Check sheet for the modelled part. Datum: model origin and axes. Units: mm. A direction names the side the tool comes from. Give positions to 0.01 mm unless a question says otherwise; leave off trailing zeros. Order: outer loops, then holes, each group sorted by start corner. A loop starts at its lowest first (then second) coordinate and runs counter-clockwise, first axis right, second up. Notation, with made-up numbers: (87.25, -13.5) -> (118.25, -13.5) arc R27 cw to (118.25, 4.5) -> close; hole circle Ø1 at (74.25, 79.25). An arc over 180 degrees is marked (long way). Answer in a Markdown table with one row per item. Add a question column.
(1) Set-up check for faces 4 (the face through (1.4, 4.4, 23.7)), 5 (the face through (-7, 7, 3.1)): record each of +Z, -Z, +X, -X, +Y, -Y from which the full face is reachable in a straight line by a thin tool's end or side.
(2) Cross-section at C-C (y = -9). State how many separate pieces and enclosed holes the cut face has, then the cut area to 3 significant figures.
(3) Go/stop test with flat-tipped pins: pin 1 (4 mm diameter, centred on y = -8, z = 17, fed in from -X); pin 2 (2 mm diameter, centred on x = -6, y = 9, fed in from +Z); pin 3 (5 mm diameter, centred on x = 0.5, y = 3.5, fed in from +Z). Record where each tip stops, or that it passes through.
(4) Cross-section at B-B (z = 14.75). Record the cut outline in (x, y).
(5) Release check for a two-part mould opening along X. For faces 1 (the face through (-8.106, -6.777, 3.987)), 2 (the face through (-12.5, 0, 2)), 3 (the face through (11.3, -11.33, 2.53)) record: released by +X, released by -X, zero draft, split by the parting line, or undercut.
(6) Thickness scan on L1, parallel to X at y = 8.5, z = 2; L2, parallel to Z at x = 10.75, y = 7.75; L3, parallel to Z at x = -4.5, y = -8.25. Record the ranges inside material, lowest first. Write a range as [from, to].
(7) Cross-section at A-A (z = 3.5). Record the cut outline in (x, y), then the cut area to 3 significant figures.
```python
from build123d import *

# Parameters (mm, degrees)
SKETCH_1_W          = 25
SKETCH_1_H          = 25
SKETCH_1_R          = 7.5
EXTRUDE_1_DEPTH     = 5
SKETCH_3_OUTSIDE_W  = 34.142
SKETCH_3_OUTSIDE_H  = 34.142
SKETCH_3_OUTSIDE_R  = 16
CUT_EXTRUDE_2_DEPTH = 5
SKETCH_5_R          = 1.75
CUT_EXTRUDE_3_DEPTH = 5
SKETCH_5_3_R        = 3
SKETCH_5_3_R_2      = 1.75
CUT_EXTRUDE_4_DEPTH = 3.1
CHAMFER_1_SIZE      = 0.1
SKETCH_7_R          = 7.5
SKETCH_7_R_2        = 6.9
EXTRUDE_2_DEPTH     = 24
FILLET_1_R          = 0.2
CHAMFER_2_SIZE      = 0.1
FILLET_2_R          = 0.1


with BuildPart() as part:
    # Sketch 1 → Extrude 1 (new body)
    with BuildSketch(Plane.XY):
        Rectangle(SKETCH_1_W, SKETCH_1_H)
        Circle(SKETCH_1_R, mode=Mode.SUBTRACT)
    extrude(amount=EXTRUDE_1_DEPTH)

    # Sketch 3 outside → Cut-Extrude 2 (cut)
    with BuildSketch(Plane.XY.offset(5)):
        Rectangle(SKETCH_3_OUTSIDE_W, SKETCH_3_OUTSIDE_H)
        Circle(SKETCH_3_OUTSIDE_R, mode=Mode.SUBTRACT)
    extrude(amount=-CUT_EXTRUDE_2_DEPTH, mode=Mode.SUBTRACT)

    # Sketch 5 → Cut-Extrude 3 (cut)
    with BuildSketch(Plane.XY):
        with Locations(Location((-8.485281374, 8.485281374, 0), (0, 0, 180))):  # turned: the seam where the file's is
            Circle(SKETCH_5_R)
        with Locations(Location((-8.485281374, -8.485281374, 0), (0, 0, 180))):  # turned: the seam where the file's is
            Circle(SKETCH_5_R)
        with Locations(Location((8.485281374, -8.485281374, 0), (0, 0, 180))):  # turned: the seam where the file's is
            Circle(SKETCH_5_R)
        with Locations(Location((8.485281374, 8.485281374, 0), (0, 0, 180))):  # turned: the seam where the file's is
            Circle(SKETCH_5_R)
    extrude(amount=CUT_EXTRUDE_3_DEPTH, mode=Mode.SUBTRACT)

    # Sketch 5_3 → Cut-Extrude 4 (cut)
    with BuildSketch(Plane.XY):
        with Locations((-8.485281374, 8.485281374)):
            Circle(SKETCH_5_3_R)
        with Locations(Location((-8.485281374, 8.485281374, 0), (0, 0, 180))):  # turned: the seam where the file's is
            Circle(SKETCH_5_3_R_2, mode=Mode.SUBTRACT)
        with Locations(Location((8.485281374, 8.485281374, 0), (0, 0, 180))):  # turned: the seam where the file's is
            Circle(SKETCH_5_3_R)
        with Locations(Location((8.485281374, 8.485281374, 0), (0, 0, 180))):  # turned: the seam where the file's is
            Circle(SKETCH_5_3_R_2, mode=Mode.SUBTRACT)
        with Locations((8.485281374, -8.485281374)):
            Circle(SKETCH_5_3_R)
        with Locations(Location((8.485281374, -8.485281374, 0), (0, 0, 180))):  # turned: the seam where the file's is
            Circle(SKETCH_5_3_R_2, mode=Mode.SUBTRACT)
        with Locations(Location((-8.485281374, -8.485281374, 0), (0, 0, 180))):  # turned: the seam where the file's is
            Circle(SKETCH_5_3_R)
        with Locations(Location((-8.485281374, -8.485281374, 0), (0, 0, 180))):  # turned: the seam where the file's is
            Circle(SKETCH_5_3_R_2, mode=Mode.SUBTRACT)
    extrude(amount=CUT_EXTRUDE_4_DEPTH, mode=Mode.SUBTRACT)

    # Chamfer 1
    chamfer_1_edges = [part.edges().sort_by_distance(p)[0] for p in [
        (11.485281374, 8.485281374, 0),
        (-11.485281374, 8.485281374, 0),
        (-7.5, 0, 0),
        (-7.5, 0, 5),
        (0, -12.5, 0),
        (0, -12.5, 5),
        (-12.5, 0, 0),
        (-12.5, 0, 5),
        (0, 12.5, 0),
        (0, 12.5, 5),
        (12.5, 0, 0),
        (12.5, 0, 5),
        (11.313708499, -11.313708499, 5),
        (11.313708499, 11.313708499, 5),
        (-11.313708499, 11.313708499, 5),
        (-11.313708499, -11.313708499, 5),
        (11.313708499, 11.313708499, 0),
        (-11.313708499, 11.313708499, 0),
        (11.313708499, -11.313708499, 0),
        (-11.313708499, -11.313708499, 0),
        (10.235281374, 8.485281374, 5),
        (10.235281374, -8.485281374, 5),
        (-6.735281374, -8.485281374, 5),
        (-6.735281374, 8.485281374, 5),
        (-5.485281374, -8.485281374, 0),
        (5.485281374, -8.485281374, 0),
    ]]
    chamfer(chamfer_1_edges, length=CHAMFER_1_SIZE)

    # Sketch 7 → Extrude 2 (add)
    with BuildSketch(Plane(origin=(0, 0, 0), x_dir=(-1, 0, 0), z_dir=(0, 0, -1))):
        Circle(SKETCH_7_R)
        Circle(SKETCH_7_R_2, mode=Mode.SUBTRACT)
    extrude(amount=-EXTRUDE_2_DEPTH)

    # Fillet 1
    fillet_1_edges = [part.edges().sort_by_distance(p)[0] for p in [
        (7.5, 0, 24),
    ]]
    fillet(fillet_1_edges, radius=FILLET_1_R)

    # Chamfer 2
    chamfer_2_edges = [part.edges().sort_by_distance(p)[0] for p in [
        (6.9, 0, 24),
    ]]
    chamfer(chamfer_2_edges, length=CHAMFER_2_SIZE)

    # Sketch 8 → Revolve 1 (revolve)
    with BuildSketch(Plane(origin=(0, 0, 0), x_dir=(0, 0, -1), z_dir=(1, 0, 0)), mode=Mode.PRIVATE) as revolve_1_sk:
        Polygon((-23.5, 6.9), (-0.4, 6.9), (-0.4, 6.7), (-0.2, 6.7), (-0.2, 4.3), (0, 4.3), (0, 4), (-23.9, 4), (-23.9, 4.3), (-23.7, 4.3), (-23.7, 6.7), (-23.5, 6.7), align=None)
    revolve(revolve_1_sk.sketch.rotate(Axis((0, 0, 0), (0, 0, 1)), 90), axis=Axis((0, 0, 0), (0, 0, 1)))  # turned: the seam where the file's is

    # Fillet 2
    fillet_2_edges = [part.edges().sort_by_distance(p)[0] for p in [
        (-9.987492178, 12.5, 2.5),
        (-12.5, 9.987492178, 2.5),
        (-12.5, -9.987492178, 2.5),
        (-9.987492178, -12.5, 2.5),
        (9.987492178, -12.5, 2.5),
        (12.5, -9.987492178, 2.5),
        (12.5, 9.987492178, 2.5),
        (9.987492178, 12.5, 2.5),
    ]]
    fillet(fillet_2_edges, radius=FILLET_2_R)


solid = part.part
```
Answer below:
| question | item | result |
|---|---|---|
| 1 | face 4 | +Z |
| 1 | face 5 | -Z |
| 2 | separate pieces | 3 |
| 2 | enclosed holes | 0 |
| 2 | area | 75.6 mm² |
| 3 | pin 1 | stops at x = -4.5 |
| 3 | pin 2 | stops at z = 5 |
| 3 | pin 3 | stops at z = 23.9 |
| 4 | outline | circle Ø15 at (0, 0); hole circle Ø8 at (0, 0) |
| 5 | face 1 | undercut |
| 5 | face 2 | released by -X |
| 5 | face 3 | released by +X |
| 6 | L1 | x = [-12.5, -11.49], [-5.49, 5.49], [11.49, 12.5] |
| 6 | L2 | z = [3.1, 5] |
| 6 | L3 | z = [0, 5] |
| 7 | outline | (-12.5, -9.95) arc R0.1 ccw to (-12.48, -10.01) arc R16 ccw to (-10.01, -12.48) arc R0.1 ccw to (-9.95, -12.5) -> (9.95, -12.5) arc R0.1 ccw to (10.01, -12.48) arc R16 ccw to (12.48, -10.01) arc R0.1 ccw to (12.5, -9.95) -> (12.5, 9.95) arc R0.1 ccw to (12.48, 10.01) arc R16 ccw to (10.01, 12.48) arc R0.1 ccw to (9.95, 12.5) -> (-9.95, 12.5) arc R0.1 ccw to (-10.01, 12.48) arc R16 ccw to (-12.48, 10.01) arc R0.1 ccw to (-12.5, 9.95) -> close; hole circle Ø3.5 at (-8.49, -8.49); hole circle Ø3.5 at (-8.49, 8.49); hole circle Ø8 at (0, 0); hole circle Ø3.5 at (8.49, -8.49); hole circle Ø3.5 at (8.49, 8.49) |
| 7 | area | 525 mm² |
